```python
from build123d import *

# Parameters (mm, degrees)
SKETCH1_R                    = 41.275
BOSS_EXTRUDE1_DEPTH          = 2.794
SKETCH2_R                    = 42.545
BOSS_EXTRUDE2_DEPTH          = 134.62
BOSS_EXTRUDE3_DEPTH          = 4.7625
CHAMFER1_SIZE                = 0.79375
CIRPATTERN1_COUNT            = 7
CHAMFER1_OF_CIRPATTERN1_SIZE = 0.79375
SKETCH4_R                    = 3.175
CUT_EXTRUDE1_DEPTH           = 9.525
SKETCH5_R                    = 6.731
BOSS_EXTRUDE4_DEPTH          = 15.24
FILLET1_R                    = 19.05
SKETCH6_W                    = 82.55
SKETCH6_H                    = 48.514
SKETCH6_R                    = 6.35
BOSS_EXTRUDE5_DEPTH          = 44.704
FILLET2_R                    = 3.175
FILLET3_R                    = 1.5875
SKETCH7_R                    = 12.7
BOSS_EXTRUDE6_DEPTH          = 50.8
F_7_16_20_TAPPED_HOLE1_D     = 9.92124
F_7_16_20_TAPPED_HOLE1_DEPTH = 28.702
F_7_16_20_TAPPED_HOLE1_TIP   = 2.980641204


with BuildPart() as part:
    # Sketch1 → Boss-Extrude1 (new body)
    with BuildSketch(Plane(origin=(0, 0, 0), x_dir=(1, 0, 0), z_dir=(0, 1, 0))):
        Circle(SKETCH1_R)
    extrude(amount=BOSS_EXTRUDE1_DEPTH)

    # Sketch2 → Boss-Extrude2 (add)
    with BuildSketch(Plane(origin=(0, 0, 0), x_dir=(1, 0, 0), z_dir=(0, 1, 0))):
        Circle(SKETCH2_R)
    extrude(amount=-BOSS_EXTRUDE2_DEPTH)

    # Sketch3 → Boss-Extrude3 (add)
    with BuildSketch(Plane.XZ.offset(134.62)):
        Polygon((2.749630657, -36.675591008), (5.499261314, -31.913091008), (2.749630657, -27.150591008), (-2.749630657, -27.150591008), (-5.499261314, -31.913091008), (-2.749630657, -36.675591008), align=None)
    boss_extrude3 = extrude(amount=BOSS_EXTRUDE3_DEPTH)

    # Chamfer1
    chamfer1_edges = [part.edges().sort_by_distance(p)[0] for p in [
        (0, -139.3825, -36.675591008),
        (4.124445986, -139.3825, -34.294341008),
        (4.124445986, -139.3825, -29.531841008),
        (0, -139.3825, -27.150591008),
        (-4.124445986, -139.3825, -29.531841008),
        (-4.124445986, -139.3825, -34.294341008),
    ]]
    chamfer(chamfer1_edges, length=CHAMFER1_SIZE)

    # CirPattern1: Boss-Extrude3 ×7 about axis
    cirpattern1_axis = Axis((0, 0, 0), (0, 1, 0))
    for i in range(1, CIRPATTERN1_COUNT):
        add(boss_extrude3.rotate(cirpattern1_axis, i * 360 / CIRPATTERN1_COUNT))

    # Chamfer1 of CirPattern1
    chamfer1_of_cirpattern1_edges = [part.edges().sort_by_distance(p)[0] for p in [
        (-28.674131688, -139.3825, -22.86685697),
        (-24.24084546, -139.3825, -24.606793599),
        (-20.517373025, -139.3825, -21.637423418),
        (-21.227186817, -139.3825, -16.928116608),
        (-25.660473045, -139.3825, -15.188179979),
        (-29.383945481, -139.3825, -18.15755016),
        (-35.756057369, -139.3825, 8.161086764),
        (-34.352285851, -139.3825, 3.610171277),
        (-29.709191669, -139.3825, 2.550415329),
        (-26.469869006, -139.3825, 6.041574868),
        (-27.873640524, -139.3825, 10.592490356),
        (-32.516734705, -139.3825, 11.652246304),
        (-15.912942561, -139.3825, 33.04356571),
        (-18.595754337, -139.3825, 29.108603547),
        (-16.52938303, -139.3825, 24.817739314),
        (-11.780199946, -139.3825, 24.461837243),
        (-9.097388169, -139.3825, 28.396799406),
        (-11.163759477, -139.3825, 32.687663639),
        (15.912942561, -139.3825, 33.04356571),
        (11.163759477, -139.3825, 32.687663639),
        (9.097388169, -139.3825, 28.396799406),
        (11.780199946, -139.3825, 24.461837243),
        (16.52938303, -139.3825, 24.817739314),
        (18.595754337, -139.3825, 29.108603547),
        (35.756057369, -139.3825, 8.161086764),
        (32.516734705, -139.3825, 11.652246304),
        (27.873640524, -139.3825, 10.592490356),
        (26.469869006, -139.3825, 6.041574868),
        (29.709191669, -139.3825, 2.550415329),
        (34.352285851, -139.3825, 3.610171277),
        (28.674131688, -139.3825, -22.86685697),
        (29.383945481, -139.3825, -18.15755016),
        (25.660473045, -139.3825, -15.188179979),
        (21.227186817, -139.3825, -16.928116608),
        (20.517373025, -139.3825, -21.637423418),
        (24.24084546, -139.3825, -24.606793599),
    ]]
    chamfer(chamfer1_of_cirpattern1_edges, length=CHAMFER1_OF_CIRPATTERN1_SIZE)

    # Sketch4 → Cut-Extrude1 (cut)
    with BuildSketch(Plane.XZ.offset(134.62)):
        Circle(SKETCH4_R)
    extrude(amount=-CUT_EXTRUDE1_DEPTH, mode=Mode.SUBTRACT)

    # Sketch5 → Boss-Extrude4 (add)
    with BuildSketch(Plane(origin=(0, 0, 0), x_dir=(1, 0, 0), z_dir=(0, 1, 0))):
        with BuildLine():
            Line((-65.659, 19.006724542), (-65.659, -19.006724542))
            Line((-65.659, -19.006724542), (-29.591473914, -38.283762101))
            ThreePointArc((-29.591473914, -38.283762101), (0, -48.387), (29.591473914, -38.283762101))
            Line((29.591473914, -38.283762101), (65.659, -19.006724542))
            Line((65.659, -19.006724542), (65.659, 19.006724542))
            Line((65.659, 19.006724542), (29.591473914, 38.283762101))
            ThreePointArc((29.591473914, 38.283762101), (0, 48.387), (-29.591473914, 38.283762101))
            Line((-29.591473914, 38.283762101), (-65.659, 19.006724542))
        make_face()
        with Locations((-53.213, 0)):
            Circle(SKETCH5_R, mode=Mode.SUBTRACT)
        with Locations((53.213, 0)):
            Circle(SKETCH5_R, mode=Mode.SUBTRACT)
    extrude(amount=-BOSS_EXTRUDE4_DEPTH)

    # Fillet1
    fillet1_edges = [part.edges().sort_by_distance(p)[0] for p in [
        (-65.659, -7.62, -19.006724542),
        (-29.591473914, -7.62, -38.283762101),
        (29.591473914, -7.62, -38.283762101),
        (65.659, -7.62, -19.006724542),
        (65.659, -7.62, 19.006724542),
        (29.591473914, -7.62, 38.283762101),
        (-29.591473914, -7.62, 38.283762101),
        (-65.659, -7.62, 19.006724542),
    ]]
    fillet(fillet1_edges, radius=FILLET1_R)

    # Sketch6 → Boss-Extrude5 (add)
    with BuildSketch(Plane.XY):
        with Locations((0, -42.672)):
            Rectangle(SKETCH6_W, SKETCH6_H)
        with Locations((22.86, -42.672)):
            Circle(SKETCH6_R, mode=Mode.SUBTRACT)
        with Locations((-22.86, -42.672)):
            Circle(SKETCH6_R, mode=Mode.SUBTRACT)
    extrude(amount=-BOSS_EXTRUDE5_DEPTH)

    # Fillet2
    fillet2_edges = [part.edges().sort_by_distance(p)[0] for p in [
        (41.275, -18.415, -27.510764387),
        (41.275, -66.929, -27.510764387),
        (-41.275, -66.929, -27.510764387),
        (-41.275, -18.415, -27.510764387),
    ]]
    fillet(fillet2_edges, radius=FILLET2_R)

    # Fillet3
    fillet3_edges = [part.edges().sort_by_distance(p)[0] for p in [
        (41.275, -42.672, -44.704),
        (0, -18.415, -44.704),
        (0, -66.929, -44.704),
        (-41.275, -42.672, -44.704),
        (40.34506403, -65.99906403, -44.704),
        (-40.34506403, -65.99906403, -44.704),
        (-40.34506403, -19.34493597, -44.704),
        (40.34506403, -19.34493597, -44.704),
    ]]
    fillet(fillet3_edges, radius=FILLET3_R)

    # Sketch7 → Boss-Extrude6 (add)
    with BuildSketch(Plane(origin=(0, 2.794, 0), x_dir=(-1, 0, 0), z_dir=(0, 1, 0))):
        Circle(SKETCH7_R)
    extrude(amount=BOSS_EXTRUDE6_DEPTH)

    # Sketch8 → 1_2 NPT Tapped Hole1 (revolve, cut)
    with BuildSketch(Plane(origin=(22.86, -42.672, -44.704), x_dir=(0, 1, 0), z_dir=(1, 0, 0))):
        Polygon((0, 0), (0, 28.478543693), (8.9281, 23.114), (8.9281, 13.462), (9.479726792, 13.462), (9.8827971, 0), align=None)
    revolve(axis=Axis((22.86, -42.672, -51.054), (0, 0, 1)), mode=Mode.SUBTRACT)

    # Sketch10 → 1_2 NPT Tapped Hole2 (revolve, cut)
    with BuildSketch(Plane(origin=(-22.86, -42.672, -44.704), x_dir=(0, 1, 0), z_dir=(1, 0, 0))):
        Polygon((0, 0), (0, 28.478543693), (8.9281, 23.114), (8.9281, 13.462), (9.479726792, 13.462), (9.8827971, 0), align=None)
    revolve(axis=Axis((-22.86, -42.672, -51.054), (0, 0, 1)), mode=Mode.SUBTRACT)

    # 7_16-20 Tapped Hole1
    with Locations(Plane.XZ.offset(134.62)):
        with Locations((0, 0)):
            Hole(F_7_16_20_TAPPED_HOLE1_D / 2, depth=F_7_16_20_TAPPED_HOLE1_DEPTH)
            with Locations((0, 0, -(F_7_16_20_TAPPED_HOLE1_DEPTH + F_7_16_20_TAPPED_HOLE1_TIP / 2))):  # 118° drill point
                Cone(0, F_7_16_20_TAPPED_HOLE1_D / 2, F_7_16_20_TAPPED_HOLE1_TIP, mode=Mode.SUBTRACT)


solid = part.part
```
Geometry: final body of the model. Coordinates: model frame, mm. A direction names the side the tool comes from. Round coordinates to 2 decimals unless told otherwise and drop trailing zeros. Write each loop counter-clockwise with the first axis right and the second up, starting at its lowest first coordinate (ties: lowest second). Pieces come first, ordered by that corner, then holes.
Item 1: Set-up query: faces 1 (the face through (-29.37, -136.58, -18.12)), 2 (the face through (-5.8, -18.415, -42.6)), 3 (the face through (26.46, -136.58, 6.08)), 4 (the face through (32.55, -136.58, 11.64)). Return all of +Z, -Z, +X, -X, +Y, -Y with unobstructed straight access to the full face (end or side cutting, diameter ignored); none if empty.
Item 2: Section query D-D (y = -95). Return loops of the section in (x, z) (3 decimals).
Item 3: Pin query (flat end, axial travel): P1, Ø23, axis at x = 22.86, y = -42.672, coming from the +Z side; P2, Ø1, axis at x = -39.5, z = 15.5, coming from the +Y side; P3, Ø6, axis at y = -85, z = 13.5, coming from the +X side; P4, Ø11, axis at x = 53.213, z = 0, coming from the -Y side. Return the tip coordinate at first contact, or that it passes through.
Item 4: Section query C-C (y = -26.5). Return loops of the section in (x, z) (1 decimal), plus the area to 3 significant figures.
Item 5: Section query B-B (y = -125.5). Return loops of the section in (x, z) (3 decimals).
Item 6: Material intervals for L1, parallel to Z at x = 0, y = -124 (3 decimals); L2, parallel to X at y = -10.5, z = 0, sorted ascending.
Item 7: Mould query, pull axis X, two halves, no side actions, for faces 5 (the face through (-27.85, -136.58, 10.57)), 6 (the face through (-35.747, -136.577, 8.199)), 7 (the face through (-11.132, -136.577, 32.666)), 8 (the face through (4.105, -136.577, -34.328)). Classes: +X half, -X half, draft (parallel to the pull), parting line (faces both ways), or undercut.
Item 8: Section query A-A (y = -6). Return loops of the section in (x, z).
Completed:
1. face 1: -X, -Y
1. face 2: -Z
1. face 3: -Y
1. face 4: +Z, +X, -Y
2. outline: circle Ø85.09 at (0, 0)
3. P1: stops at z = 41
3. P2: stops at y = 0
3. P3: stops at x = 41.23
3. P4: passes through
4. outline: (-41.3, -43.1) arc R1.6 ccw to (-39.7, -44.7) - (39.7, -44.7) arc R1.6 ccw to (41.3, -43.1) - (41.3, -10.3) arc R42.5 ccw (long way) to (-41.3, -10.3) - close
4. area: 6,550 mm2
5. outline: circle Ø85.09 at (0, 0); hole circle Ø9.921 at (0, 0)
6. L1: z = -42.545 to -4.961, 4.961 to 42.545
6. L2: x = -65.66 to -59.94, -46.48 to 46.48, 59.94 to 65.66
7. face 5: undercut
7. face 6: -X half
7. face 7: undercut
7. face 8: +X half
8. outline: (-65.66, -7.59) arc R19.05 ccw to (-55.59, -24.39) - (-30.88, -37.59) arc R19.05 cw to (-28.6, -39.03) arc R48.39 ccw to (28.6, -39.03) arc R19.05 cw to (30.88, -37.59) - (55.59, -24.39) arc R19.05 ccw to (65.66, -7.59) - (65.66, 7.59) arc R19.05 ccw to (55.59, 24.39) - (30.88, 37.59) arc R19.05 cw to (28.6, 39.03) arc R48.39 ccw to (-28.6, 39.03) arc R19.05 cw to (-30.88, 37.59) - (-55.59, 24.39) arc R19.05 ccw to (-65.66, 7.59) - close; hole circle Ø13.46 at (-53.21, 0); hole circle Ø13.46 at (53.21, 0)
